from build123d import *

# Parameters (mm, degrees)
F0_R     = 5.08
F1_DEPTH = 12.7
F3_D     = 13.4874
F4_W     = 6.35
F4_H     = 31.75
F5_DEPTH = 50.8


with BuildPart() as f1:
    # F0 (on Front) → F1 (new body, symmetric)
    with BuildSketch(Plane.XZ):
        with BuildLine():
            Line((20.828, -68.072), (20.828, 34.544))
            ThreePointArc((20.828, 34.544), (24.547744, 43.524256), (33.528, 47.244))
            Line((33.528, 47.244), (98.2345, 47.244))
            Line((98.2345, 47.244), (98.2345, 88.9))
            Line((98.2345, 88.9), (20.828, 88.9))
            ThreePointArc((20.828, 88.9), (-8.62724, 76.69924), (-20.828, 47.244))
            Line((-20.828, 47.244), (-20.828, -62.811488))
            ThreePointArc((-20.828, -62.811488), (-19.86127, -67.671567), (-17.108256, -71.791744))
            Line((-17.108256, -71.791744), (0, -88.9))
            ThreePointArc((0, -88.9), (14.72762, -82.79962), (20.828, -68.072))
        make_face()
        with Locations((10.414, -68.072)):
            Circle(F0_R, mode=Mode.SUBTRACT)
    extrude(amount=F1_DEPTH, both=True)

    # F3 (through all)
    with Locations(Plane(origin=(0, 0, 0), x_dir=(1, 0, 0), z_dir=(0, 0, -1))):
        with Locations((83.947, 0)):
            Hole(F3_D / 2)

    # F4 (on Right) → F5 (cut, symmetric)
    with BuildSketch(Plane.YZ):
        with Locations((3.175, -73.025)):
            Rectangle(F4_W, F4_H)
        with Locations((-3.175, -73.025)):
            Rectangle(F4_W, F4_H)
    extrude(amount=F5_DEPTH, both=True, mode=Mode.SUBTRACT)


solid = f1.part
Work out the finished part from the listing and answer in its coordinate system (mm). A direction names the side the tool comes from. Give positions to 0.01 mm unless a question says otherwise; leave off trailing zeros. Order: outer loops, then holes, each group sorted by start corner. A loop starts at its lowest first (then second) coordinate and runs counter-clockwise, first axis right, second up. Notation, with made-up numbers: M -25,8 L 18,8 A19 ccw 18,16 Z; hole C 45,-3.75 d5. An arc over 180 degrees is marked long. Return JSON: item names as keys, results as strings.
Q1. Each of these flat-tipped pins is pushed along its axis until it touches: pin 1 (6 mm diameter, centred on x = 17, y = -8.5, fed in from +Z); pin 2 (1.5 mm diameter, centred on x = 55, y = -3.5, fed in from -Z); pin 3 (2 mm diameter, centred on x = 12.5, y = 8.5, fed in from -Z); pin 4 (13 mm diameter, centred on x = 10.414, z = -68.072, fed in from +Y). Where does it stop, or does it pass through?
Answer below:
{"pin 1": "stops at z = 88.89", "pin 2": "stops at z = 47.24", "pin 3": "stops at z = -85.44", "pin 4": "stops at y = 12.7"}
Q2. Find section A-A, the plane y = 0. Write down the section's boundary in (x, z).
Answer below:
{"outline": "M -20.83,-57.15 L 20.83,-57.15 L 20.83,34.54 A12.7 cw 33.53,47.24 L 77.2,47.24 L 77.2,88.9 L 20.83,88.9 A41.66 ccw -20.83,47.24 Z; M 90.69,47.24 L 98.23,47.24 L 98.23,88.9 L 90.69,88.9 Z"}
Q3. Find section C-C, the plane x = -10. Write down the section's boundary in (y, z), and give its area (3 significant figures).
Answer below:
{"outline": "M -12.7,-78.9 L -6.35,-78.9 L -6.35,-57.15 L 6.35,-57.15 L 6.35,-78.9 L 12.7,-78.9 L 12.7,75.26 L -12.7,75.26 Z", "area": "3,640 mm^2"}
Q4. Find section B-B, the plane y = 9. Write down the section's boundary in (x, z).
Answer below:
{"outline": "M -20.83,-62.81 A12.7 ccw -17.11,-71.79 L 0,-88.9 A20.83 ccw 20.83,-68.07 L 20.83,34.54 A12.7 cw 33.53,47.24 L 98.23,47.24 L 98.23,88.9 L 20.83,88.9 A41.66 ccw -20.83,47.24 Z; hole C 10.41,-68.07 d10.16"}
Q5. Which of the six approach directions +Z, -Z, +X, -X, +Y, -Y give full straight-line access (tool end or side, diameter ignored) to faces 1 (the face through (65, 0, 47.244)), 2 (the face through (-8.302, -0.178, 77.021)), 3 (the face through (0, 6.35, -70))?
Answer below:
{"face 1": "-Z, +X, +Y, -Y", "face 2": "+Z, -X, +Y, -Y", "face 3": "-Z, +X, -X"}
Q6. The mould has two halves that part along Y. Classify faces 4 (the face through (14.565, 9.481, -82.961)), 5 (the face through (11, 12.7, 21)), 6 (the face through (0, 0, -57.15)): pulls with the +Y half, pulls with the -Y half, needs draft (parallel to the pull), parting line crosses it, or undercut.
Answer below:
{"face 4": "needs draft", "face 5": "pulls with the +Y half", "face 6": "undercut"}
Q7. Find the intervals of material crossed by line 1 along Z through (x, y) = (86, 9.5); line 2 along X through (y, z) = (-4.25, 24); line 3 along Y through (x, z) = (82.5, 63.5), in increasing order. Write a range as [from, to].
Answer below:
{"line 1": "z = [47.24, 88.9]", "line 2": "x = [-20.83, 20.83]", "line 3": "y = [-12.7, -6.59], [6.59, 12.7]"}
Q8. Find section D-D, the plane z = -51. Write down the section's boundary in (x, y).
Answer below:
{"outline": "M -20.83,-12.7 L 20.83,-12.7 L 20.83,12.7 L -20.83,12.7 Z"}
